Design review of the part built by this model. Coordinates are the model's own, in mm. Give positions to 0.01 mm unless a question says otherwise; leave off trailing zeros. Order: outer loops, then holes, each group sorted by start corner. A loop starts at its lowest first (then second) coordinate and runs counter-clockwise, first axis right, second up.
```python
from build123d import *

# Parameters (mm, degrees)
F0_W     = 100
F0_H     = 100
F1_DEPTH = 100
F2_R     = 5
F3_DEPTH = 100


with BuildPart() as f1:
    # F0 (on Right) → F1 (new body)
    with BuildSketch(Plane.YZ):
        with Locations((50, 50)):
            Rectangle(F0_W, F0_H)
    extrude(amount=F1_DEPTH)

    # F2 (on face) → F3 (cut)
    with BuildSketch(Plane.XY.offset(100)):
        with Locations((15, 25)):
            Circle(F2_R)
        with Locations((142.386928, 39.02828)):
            Circle(F2_R)
        with Locations((15, 50)):
            Circle(F2_R)
        with Locations((15, 75)):
            Circle(F2_R)
    extrude(amount=-F3_DEPTH, mode=Mode.SUBTRACT)


solid = f1.part
```
1. Take a section at A-A (x = 15). State the section outline as (y, z) points.
Recorded:
outline: (0, 0) - (20, 0) - (20, 100) - (0, 100) - close; (30, 0) - (45, 0) - (45, 100) - (30, 100) - close; (55, 0) - (70, 0) - (70, 100) - (55, 100) - close; (80, 0) - (100, 0) - (100, 100) - (80, 100) - close
2. Draft analysis for pull direction X (two halves, no side actions). For faces 1 (the face through (17.307, 20.564, 50.7)), 2 (the face through (49, 0, 49)), 3 (the face through (100, 49, 51)), state which applies: pulls with the +X half, pulls with the -X half, needs draft (parallel to the pull), parting line crosses it, or undercut.
Recorded:
face 1: undercut
face 2: needs draft
face 3: pulls with the +X half
3. For line 1 along Y through (x, z) = (15, 63.5), list the stretches that pass through material, from the lowest coordinate up.
Recorded:
line 1: y = 0 to 20, 30 to 45, 55 to 70, 80 to 100
4. Take a section at B-B (y = 75). State the section outline as (x, z) points, then the cut area to 3 significant figures.
Recorded:
outline: (0, 0) - (10, 0) - (10, 100) - (0, 100) - close; (20, 0) - (100, 0) - (100, 100) - (20, 100) - close
area: 9,000 mm2
5. Take a section at C-C (z = 31). State the section outline as (x, y) points, then the cut area to 3 significant figures.
Recorded:
outline: (0, 0) - (100, 0) - (100, 100) - (0, 100) - close; hole circle Ø10 at (15, 25); hole circle Ø10 at (15, 50); hole circle Ø10 at (15, 75)
area: 9,760 mm2
